Input: part model. Units: mm. Frame: model coordinates. Give positions to 0.01 mm unless a question says otherwise; leave off trailing zeros. Loops run counter-clockwise (first coordinate to the right, second up) from the corner with the lowest first, then second, coordinate; pieces in that order, holes last. Notation, with made-up numbers: M 86.25,87 L 124.25,87 A21 cw 124.25,114 Z; hole C -28.75,67 d3. An arc over 180 degrees is marked long. Use a Markdown table: item, result. Add a question column.
from build123d import *

# Parameters (mm, degrees)
IZIM2_R                     = 35
IZIM2_R_2                   = 1.5
Y_KSEKLIK_EKSTR_ZYON1_DEPTH = 0.5


with BuildPart() as part:
    # Çizim2 → Yükseklik-Ekstrüzyon1 (new body)
    with BuildSketch(Plane.XY):
        Circle(IZIM2_R)
        with Locations((-15.31013221, -26.517926859)):
            Circle(IZIM2_R_2, mode=Mode.SUBTRACT)
        with Locations((30.62026442, 0)):
            Circle(IZIM2_R_2, mode=Mode.SUBTRACT)
        with Locations((-15.31013221, 26.517926859)):
            Circle(IZIM2_R_2, mode=Mode.SUBTRACT)
        with Locations((15.31013221, 26.517926859)):
            Circle(IZIM2_R_2, mode=Mode.SUBTRACT)
        with Locations((15.31013221, -26.517926859)):
            Circle(IZIM2_R_2, mode=Mode.SUBTRACT)
        with Locations((-30.62026442, 0)):
            Circle(IZIM2_R_2, mode=Mode.SUBTRACT)
        with BuildLine():
            Line((-15.110106202, 10.455874691), (-15.976131606, 10.955874691))
            Line((-15.976131606, 10.955874691), (-13.59215701, 17.085039816))
            Line((-13.59215701, 17.085039816), (-15.806258625, 21.250103325))
            ThreePointArc((-15.806258625, 21.250103325), (-18.402735589, 22.841478137), (-21.05330993, 21.341937514))
            Line((-21.05330993, 21.341937514), (-29.009315019, 7.561732477))
            ThreePointArc((-29.009315019, 7.561732477), (-28.982668121, 4.516497451), (-26.306258625, 3.063569846))
            Line((-26.306258625, 3.063569846), (-21.59215701, 3.228633355))
            Line((-21.59215701, 3.228633355), (-17.476131606, 8.35779848))
            Line((-17.476131606, 8.35779848), (-16.610106202, 7.85779848))
            ThreePointArc((-16.610106202, 7.85779848), (-18.375, 0), (-16.610106202, -7.85779848))
            Line((-16.610106202, -7.85779848), (-17.476131606, -8.35779848))
            Line((-17.476131606, -8.35779848), (-21.59215701, -3.228633355))
            Line((-21.59215701, -3.228633355), (-26.306258625, -3.063569846))
            ThreePointArc((-26.306258625, -3.063569846), (-28.982668121, -4.516497451), (-29.009315018, -7.561732476))
            Line((-29.009315018, -7.561732476), (-21.05330993, -21.341937514))
            ThreePointArc((-21.05330993, -21.341937514), (-18.402735589, -22.841478137), (-15.806258625, -21.250103325))
            Line((-15.806258625, -21.250103325), (-13.59215701, -17.085039816))
            Line((-13.59215701, -17.085039816), (-15.976131606, -10.955874691))
            Line((-15.976131606, -10.955874691), (-15.110106202, -10.455874691))
            ThreePointArc((-15.110106202, -10.455874691), (-9.1875, -15.913216795), (-1.5, -18.313673171))
            Line((-1.5, -18.313673171), (-1.5, -19.313673171))
            Line((-1.5, -19.313673171), (-8, -20.313673171))
            Line((-8, -20.313673171), (-10.5, -24.313673171))
            ThreePointArc((-10.5, -24.313673171), (-10.579932532, -27.357975588), (-7.956005088, -28.903669991))
            Line((-7.956005088, -28.903669991), (7.956005088, -28.903669991))
            ThreePointArc((7.956005088, -28.903669991), (10.579932532, -27.357975588), (10.5, -24.313673171))
            Line((10.5, -24.313673171), (8, -20.313673171))
            Line((8, -20.313673171), (1.5, -19.313673171))
            Line((1.5, -19.313673171), (1.5, -18.313673171))
            ThreePointArc((1.5, -18.313673171), (9.1875, -15.913216795), (15.110106202, -10.455874691))
            Line((15.110106202, -10.455874691), (15.976131606, -10.955874691))
            Line((15.976131606, -10.955874691), (13.59215701, -17.085039816))
            Line((13.59215701, -17.085039816), (15.806258625, -21.250103325))
            ThreePointArc((15.806258625, -21.250103325), (18.402735589, -22.841478137), (21.05330993, -21.341937514))
            Line((21.05330993, -21.341937514), (29.009315019, -7.561732476))
            ThreePointArc((29.009315019, -7.561732476), (28.982668121, -4.516497451), (26.306258625, -3.063569846))
            Line((26.306258625, -3.063569846), (21.59215701, -3.228633355))
            Line((21.59215701, -3.228633355), (17.476131606, -8.35779848))
            Line((17.476131606, -8.35779848), (16.610106202, -7.85779848))
            ThreePointArc((16.610106202, -7.85779848), (18.375, 0), (16.610106202, 7.85779848))
            Line((16.610106202, 7.85779848), (17.476131606, 8.35779848))
            Line((17.476131606, 8.35779848), (21.59215701, 3.228633355))
            Line((21.59215701, 3.228633355), (26.306258625, 3.063569846))
            ThreePointArc((26.306258625, 3.063569846), (28.982668121, 4.516497451), (29.009315018, 7.561732476))
            Line((29.009315018, 7.561732476), (21.05330993, 21.341937514))
            ThreePointArc((21.05330993, 21.341937514), (18.402735589, 22.841478137), (15.806258625, 21.250103325))
            Line((15.806258625, 21.250103325), (13.59215701, 17.085039816))
            Line((13.59215701, 17.085039816), (15.976131606, 10.955874691))
            Line((15.976131606, 10.955874691), (15.110106202, 10.455874691))
            ThreePointArc((15.110106202, 10.455874691), (9.1875, 15.913216795), (1.5, 18.313673171))
            Line((1.5, 18.313673171), (1.5, 19.313673171))
            Line((1.5, 19.313673171), (8, 20.313673171))
            Line((8, 20.313673171), (10.5, 24.313673171))
            ThreePointArc((10.5, 24.313673171), (10.579932532, 27.357975588), (7.956005088, 28.903669991))
            Line((7.956005088, 28.903669991), (-7.956005088, 28.903669991))
            ThreePointArc((-7.956005088, 28.903669991), (-10.579932532, 27.357975588), (-10.5, 24.313673171))
            Line((-10.5, 24.313673171), (-8, 20.313673171))
            Line((-8, 20.313673171), (-1.5, 19.313673171))
            Line((-1.5, 19.313673171), (-1.5, 18.313673171))
            ThreePointArc((-1.5, 18.313673171), (-9.1875, 15.913216795), (-15.110106202, 10.455874691))
        make_face(mode=Mode.SUBTRACT)
    extrude(amount=Y_KSEKLIK_EKSTR_ZYON1_DEPTH)


solid = part.part
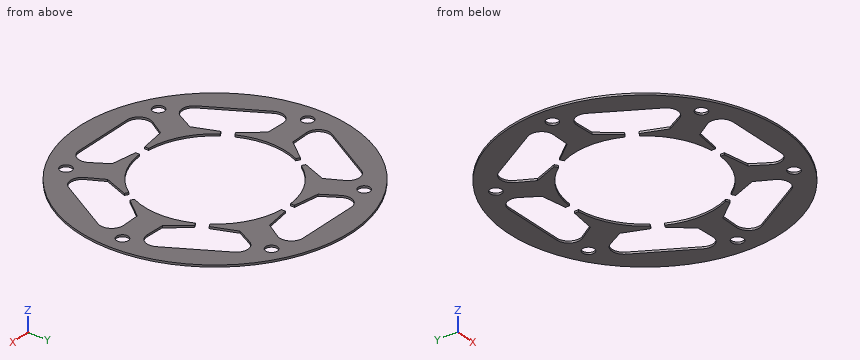
1) Section query A-A, the plane x = 0. Return the cut outline in (y, z), and give its area (3 significant figures).
2) Section query D-D, the plane y = 16. Return the cut outline in (x, z), and give its area (3 significant figures).
3) Ray query, line 1 (Y direction, x = 28, z = 0.4); line 2 (Y direction, x = -5, z = 0.1); line 3 (X direction, y = 8, z = 0.1). Return the intervals inside material, ascending. Write a range as [from, to].
4) Section query C-C, the plane x = 19.5. Return the cut outline in (y, z).
5) Contact query for flat-ended pins moving along their axis: P1, Ø4, axis at x = -30.62, y = 0, coming from the +Z side; P2, Ø2.5, axis at x = -15.31, y = 26.52, coming from the -Z side. Output: stop coordinate, or through.
6) Section query B-B, the plane y = 0. Return the cut outline in (x, z) (3 decimals), and give its area (3 significant figures).
Entries:
| question | item | result |
|---|---|---|
| 1 | outline | M -35,0 L -28.9,0 L -28.9,0.5 L -35,0.5 Z; M 28.9,0 L 35,0 L 35,0.5 L 28.9,0.5 Z |
| 1 | area | 6.10 mm² |
| 2 | outline | M -31.13,0 L -24.14,0 L -24.14,0.5 L -31.13,0.5 Z; M -14.01,0 L -9.04,0 L -9.04,0.5 L -14.01,0.5 Z; M 9.04,0 L 14.01,0 L 14.01,0.5 L 9.04,0.5 Z; M 24.14,0 L 31.13,0 L 31.13,0.5 L 24.14,0.5 Z |
| 2 | area | 12.0 mm² |
| 3 | line 1 | y = [-21, -9.31], [-3.52, 3.52], [9.31, 21] |
| 3 | line 2 | y = [-34.64, -28.9], [-19.85, -17.68], [17.68, 19.85], [28.9, 34.64] |
| 3 | line 3 | x = [-34.07, -28.76], [-17.76, -16.86], [16.86, 17.76], [28.76, 34.07] |
| 4 | outline | M -29.06,0 L -22.65,0 L -22.65,0.5 L -29.06,0.5 Z; M -5.84,0 L 5.84,0 L 5.84,0.5 L -5.84,0.5 Z; M 22.65,0 L 29.06,0 L 29.06,0.5 L 22.65,0.5 Z |
| 5 | P1 | stops at z = 0.5 |
| 5 | P2 | passes through |
| 6 | outline | M -35,0 L -32.12,0 L -32.12,0.5 L -35,0.5 Z; M -29.12,0 L -18.375,0 L -18.375,0.5 L -29.12,0.5 Z; M 18.375,0 L 29.12,0 L 29.12,0.5 L 18.375,0.5 Z; M 32.12,0 L 35,0 L 35,0.5 L 32.12,0.5 Z |
| 6 | area | 13.6 mm² |
